from build123d import *

# Parameters (mm, degrees)
SKETCH1_W           = 60
SKETCH1_H           = 40
BOSS_EXTRUDE1_DEPTH = 20
SKETCH2_R           = 10
BOSS_EXTRUDE2_DEPTH = 20
SKETCH4_W           = 20
SKETCH4_H           = 10
CUT_EXTRUDE1_DEPTH  = 75.833147735


with BuildPart() as part:
    # Sketch1 → Boss-Extrude1 (new body)
    with BuildSketch(Plane(origin=(0, 0, 0), x_dir=(1, 0, 0), z_dir=(0, 1, 0))):
        Rectangle(SKETCH1_W, SKETCH1_H)
    extrude(amount=BOSS_EXTRUDE1_DEPTH)

    # Sketch2 → Boss-Extrude2 (add)
    with BuildSketch(Plane(origin=(0, 20, 0), x_dir=(1, 0, 0), z_dir=(0, 1, 0))):
        with Locations(Location((0, 0, 0), (0, 0, 270))):
            Circle(SKETCH2_R)
    extrude(amount=BOSS_EXTRUDE2_DEPTH)

    # Sketch4 → Cut-Extrude1 (cut, through all)
    with BuildSketch(Plane.ZY.offset(30)):
        with Locations((0, 5)):
            Rectangle(SKETCH4_W, SKETCH4_H)
    extrude(amount=-CUT_EXTRUDE1_DEPTH, mode=Mode.SUBTRACT)


solid = part.part
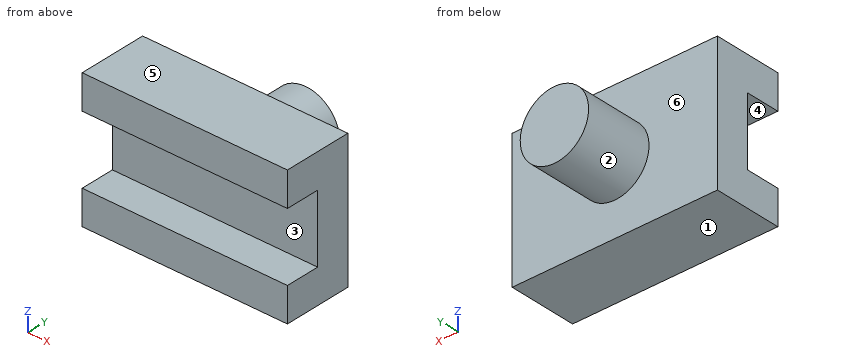
Source: CAD feature listing. Evaluate the final solid. Frame: model axes, mm. Face numbers are marked on the shaded views. A direction names the side the tool comes from. Round coordinates to 2 decimals unless told otherwise and drop trailing zeros. Loops run counter-clockwise (first coordinate to the right, second up) from the corner with the lowest first, then second, coordinate; pieces in that order, holes last. Notation, with made-up numbers: (-26.5, 86) -> (20.5, 86) arc R12 cw to (20.5, 109) -> close; hole circle Ø1 at (48.5, 44.25). An arc over 180 degrees is marked (long way). Answer as a JSON object with one key per item and string values. Group by question number.
Q1. Ray query, line 1 (Z direction, x = 26.5, y = 7.5); line 2 (Y direction, x = 7.5, z = 3); line 3 (Y direction, x = -8, z = -13). Return the intervals inside material, ascending. Write a range as from..to.
Q2. Contact query for flat-ended pins moving along their axis: P1, Ø12, axis at x = -6, z = -9, coming from the +Y side; P2, Ø12, axis at x = 24, z = -7, coming from the +Y side; P3, Ø1.5, axis at x = 16, z = 2, coming from the -Y side. Output: stop coordinate, or through.
Q3. Mould query, pull axis Z, two halves, no side actions, for the marked faces 4, 5 and 6. Classes: pulls with the +Z half, pulls with the -Z half, needs draft (parallel to the pull), parting line crosses it, or undercut.
Q4. Access query for the marked faces 1, 2 and 3. Directions: +Z, -Z, +X, -X, +Y, -Y. A direction counts if a zero-diameter tool reaches every point of the face in a straight line with its end or side. Return the directions, or none.
Q5. Section query C-C (z = 0). Output: boundary loops of the cut face in (x, y), plus the area to 3 significant figures.
Q6. Section query B-B (x = 0). Output: boundary loops of the cut face in (y, z), plus the area to 3 significant figures.
Q7. Section query D-D (y = 33.5). Output: boundary loops of the cut face in (x, z).
Q8. Section query A-A (y = 4). Output: boundary loops of the cut face in (x, z), plus the area to 3 significant figures.
Completed:
{
 "1": {"line 1": "-20..-10, 10..20", "line 2": "10..40", "line 3": "0..20"},
 "2": {"P1": "y = 40", "P2": "y = 20", "P3": "y = 10"},
 "3": {"face 4": "undercut", "face 5": "pulls with the +Z half", "face 6": "needs draft"},
 "4": {"face 1": "-Z, +X, -X, +Y, -Y", "face 2": "+Y", "face 3": "+X, -X, -Y"},
 "5": {"outline": "(-30, 10) -> (30, 10) -> (30, 20) -> (10, 20) -> (10, 40) -> (-10, 40) -> (-10, 20) -> (-30, 20) -> close", "area": "1,000 mm²"},
 "6": {"outline": "(0, -20) -> (20, -20) -> (20, -10) -> (40, -10) -> (40, 10) -> (20, 10) -> (20, 20) -> (0, 20) -> (0, 10) -> (10, 10) -> (10, -10) -> (0, -10) -> close", "area": "1,000 mm²"},
 "7": {"outline": "circle Ø20 at (0, 0)"},
 "8": {"outline": "(-30, -20) -> (30, -20) -> (30, -10) -> (-30, -10) -> close; (-30, 10) -> (30, 10) -> (30, 20) -> (-30, 20) -> close", "area": "1,200 mm²"}
}
